Input: part model. Units: mm. Frame: model coordinates. Coordinates: 2 decimals unless noted, no trailing zeros. Loops run counter-clockwise (first coordinate to the right, second up) from the corner with the lowest first, then second, coordinate; pieces in that order, holes last.
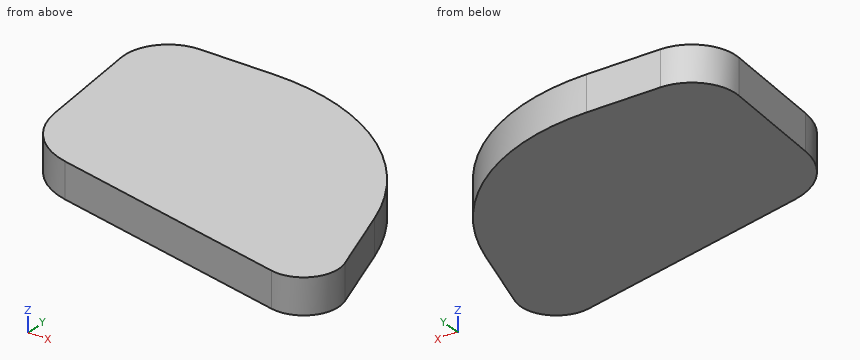
```python
from build123d import *

# Parameters (mm, degrees)
BOSS_EXTRUDE1_DEPTH = 4
SCALE1_SCALE        = 0.709677419
SCALE2_SCALE        = 1.107011


with BuildPart() as part:
    # Sketch1 → Boss-Extrude1 (new body)
    with BuildSketch(Plane.XY):
        with BuildLine():
            Line((147.518542688, 207.036750067), (155.868006274, 207.036750067))
            ThreePointArc((155.868006274, 207.036750067), (170.568083888, 202.258216832), (179.648576747, 189.749367518))
            Line((179.648576747, 189.749367518), (182.461666016, 181.075675605))
            ThreePointArc((182.461666016, 181.075675605), (181.615221362, 177.149521305), (177.786078934, 175.937570644))
            Line((177.786078934, 175.937570644), (150.012503839, 182.131679667))
            ThreePointArc((150.012503839, 182.131679667), (145.770913066, 184.629115543), (143.794281074, 189.137020178))
            Line((143.794281074, 189.137020178), (142.543783701, 201.534980175))
            ThreePointArc((142.543783701, 201.534980175), (143.809846862, 205.390192369), (147.518542688, 207.036750067))
        make_face()
    extrude(amount=BOSS_EXTRUDE1_DEPTH)


with BuildPart() as part_1:
    # Scale1: scaled about (161.61313874, 191.864088439, 2)
    add(part.part.scale(SCALE1_SCALE).moved(Location((46.919943505, 55.702477289, 0.580645161))))


with BuildPart() as part_2:
    # Scale2: scaled about (161.61313874, 191.864088439, 2)
    add(part_1.part.scale(SCALE2_SCALE).moved(Location((-17.29438359, -20.531567968, -0.214022))))


solid = part_2.part
```
Item 1: Contact query for a flat-ended pin moving along its axis: P1, Ø1.5, axis at x = 168.5, z = 1.5, coming from the +Y side. Output: stop coordinate, or through.
Result:
P1: stops at y = 200.65
Item 2: Section query B-B (y = 193). Output: boundary loops of the cut face in (x, z).
Result:
outline: (147.28, 0.43) - (174.63, 0.43) - (174.63, 3.57) - (147.28, 3.57) - close
Item 3: Line query: L1, parallel to X at y = 188, z = 0.7; L2, parallel to X at y = 185.5, z = 3.3; L3, parallel to Y at x = 152.5, z = 2.2. Output: solid intervals per line, ascending.
Result:
L1: x = 148.04 to 176.5
L2: x = 149.87 to 177.31
L3: y = 184.22 to 203.78
Item 4: Section query C-C (x = 164.5). Output: boundary loops of the cut face in (y, z).
Result:
outline: (181.54, 0.43) - (202.34, 0.43) - (202.34, 3.57) - (181.54, 3.57) - close
Item 5: Section query A-A (z = 2.05). Output: boundary loops of the cut face in (x, y), then the cut area to 3 significant figures.
Result:
outline: (146.63, 199.46) - (147.61, 189.72) arc R6.28 ccw to (152.5, 184.22) - (174.32, 179.35) arc R3.14 ccw to (177.99, 183.39) - (175.78, 190.2) arc R19.64 ccw to (157.1, 203.78) - (150.54, 203.78) arc R3.93 ccw to start
area: 557 mm2
